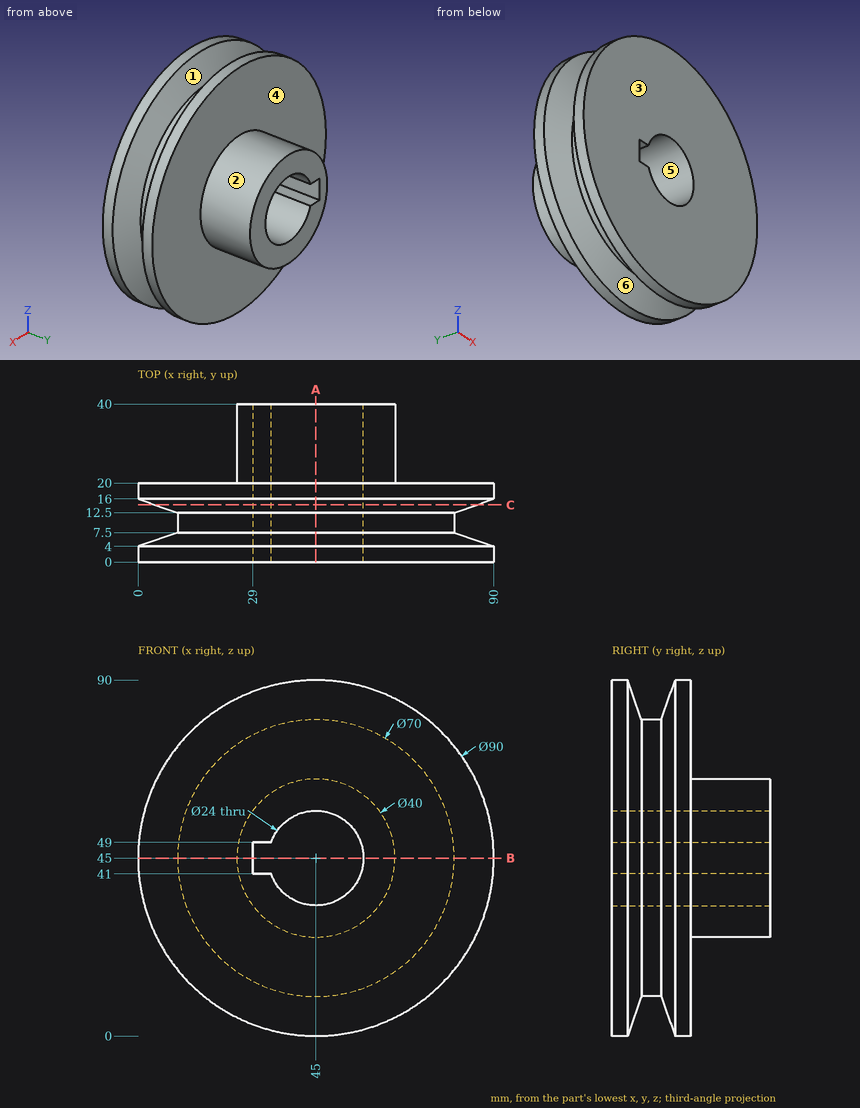
Can you work these out from the drawing? Everything is in mm from the part's minimum corner. A direction names the side the tool comes from. Give positions to 0.01 mm unless a question says otherwise; leave off trailing zeros. Order: outer loops, then holes, each group sorted by start corner. A loop starts at its lowest first (then second) coordinate and runs counter-clockwise, first axis right, second up. Notation, with made-up numbers: M -6.5,75.25 L 20.5,75.25 A13 cw 20.5,81.25 Z; hole C 12.25,-30.75 d1. An arc over 180 degrees is marked long. Use a Markdown table: item, result. Add a question column.
1. On a 3-axis mill with a long thin cutter (end or side, diameter ignored), from which of +Z, -Z, +X, -X, +Y, -Y can I reach the whole of each face in a straight line? I mean the marked faces 1, 2 and 3. Say none if no direction works.
2. Suppose I cut it at C-C (y = 14.5). List the corners of the cut face in (x, z) for me, and give its area (3 significant figures).
3. Suppose I cut it at B-B (z = 45). List the corners of the cut face in (x, y) for me.
4. For pin 1 Ø8 at (x, y) = (59, 26.5) entering from -Z; pin 2 Ø1.5 at (x, y) = (26, 27) entering from +Z; pin 3 Ø5 at (x, y) = (31.5, 30) entering from +Z, each with a flat end and sliding along its axis, tell me the tip position at first contact or that it passes through.
5. If we mould it in two halves opening along X, with no side actions, what happens to the marked faces 4, 5 and 6? For each: +X half, -X half, draft (parallel to the pull), parting line (faces both ways), or undercut.
6. I need wall thicknesses on probe 1 along Z at (x, y) = (45, 21.5); probe 2 along Z at (x, y) = (45, 17); probe 3 along X at (y, z) = (32, 45). Which ranges of each line are inside material? Lowest first, please. Write a range as from..to.
7. Suppose I cut it at A-A (x = 45). List the corners of the cut face in (y, z) for me.
Results list:
| question | item | result |
|---|---|---|
| 1 | face 1 | none |
| 1 | face 2 | +Y |
| 1 | face 3 | +Z, -Z, +X, -X, -Y |
| 2 | outline | C 45,45 d81.43; hole M 29,41 L 33.69,41 A12 ccw long 33.69,49 L 29,49 Z |
| 2 | area | 4,720 mm² |
| 3 | outline | M 0,0 L 29,0 L 29,40 L 25,40 L 25,20 L 0,20 L 0,16 L 10,12.5 L 10,7.5 L 0,4 Z; M 57,0 L 90,0 L 90,4 L 80,7.5 L 80,12.5 L 90,16 L 90,20 L 65,20 L 65,40 L 57,40 Z |
| 4 | pin 1 | stops at z = 27.68 |
| 4 | pin 2 | stops at z = 53.18 |
| 4 | pin 3 | stops at z = 61.7 |
| 5 | face 4 | draft |
| 5 | face 5 | undercut |
| 5 | face 6 | parting line |
| 6 | probe 1 | z = 25..33, 57..65 |
| 6 | probe 2 | z = 0..33, 57..90 |
| 6 | probe 3 | x = 25..29, 57..65 |
| 7 | outline | M 0,0 L 4,0 L 7.5,10 L 12.5,10 L 16,0 L 20,0 L 20,25 L 40,25 L 40,33 L 0,33 Z; M 0,57 L 40,57 L 40,65 L 20,65 L 20,90 L 16,90 L 12.5,80 L 7.5,80 L 4,90 L 0,90 Z |
